Design review of the part built by this model. Coordinates are the model's own, in mm. A direction names the side the tool comes from. Give positions to 0.01 mm unless a question says otherwise; leave off trailing zeros. Loops run counter-clockwise (first coordinate to the right, second up) from the corner with the lowest first, then second, coordinate; pieces in that order, holes last. Notation, with made-up numbers: M 2.25,68.5 L 44.25,68.5 A20 cw 44.25,72.5 Z; hole C -2,-10.5 d6. An arc over 180 degrees is marked long. Use a Markdown table: item, result. Add a question column.
(1) Add section D-D, the plane x = -16.5. Give the boundary of the cut face in (y, z).
(2) For faces 4 (the face through (-5, 12.5, 0)), 5 (the face through (78.74, 18.78, -0.17)), list the 3-axis set-ups (+Z, -Z, +X, -X, +Y, -Y) from which the entire face can be reached by the end or side of a thin tool; tool diameter is ignored.
(3) Add section B-B, the plane x = 0. Give the boundary of the cut face in (y, z), then the cut area to 3 significant figures.
(4) For probe 1 along X at (y, z) = (28.75, 0); probe 2 along Y at (x, z) = (-37.5, 6.25); probe 3 along X at (y, z) = (18, 0), list the stretches that pass through material, from the lowest coordinate up.
(5) Add section A-A, the plane z = 0. Give the boundary of the cut face in (x, y).
(6) Add section C-C, the plane y = 29.5. Give the boundary of the cut face in (x, z).
(7) Draft analysis for pull direction Z (two halves, no side actions). For faces 1 (the face through (-58.42, 6.16, 0.17)), 2 (the face through (9, 10, -7.62)), 3 (the face through (2.52, 31.84, -0.33)), state which applies: pulls with the +Z half, pulls with the -Z half, needs draft (parallel to the pull), parting line crosses it, or undercut.
(8) Insertion check: pin 1 Ø1 at (y, z) = (23, -4) entering from +X; pin 2 Ø2 at (y, z) = (7.5, 0.5) entering from -X; pin 3 Ø1 at (y, z) = (31.5, -1.5) entering from +X; pin 4 Ø4 at (y, z) = (21.5, -0.5) entering from -X. Each pin has a flat end and moves straight along its axis. Give the tip position at first contact, or say it passes through.
```python
from build123d import *

# Parameters (mm, degrees)
BOSS_EXTRUDE1_DEPTH     = 38.1
SKETCH4_R               = 2.54
CUT_EXTRUDE3_DEPTH      = 88.804680969
CUT_EXTRUDE4_DEPTH      = 6.35
CUT_EXTRUDE4_DEPTH_BACK = 6.550000108


with BuildPart() as part:
    # Sketch3 → Boss-Extrude1 (new body)
    with BuildSketch(Plane(origin=(0, 0, 0), x_dir=(1, 0, 0), z_dir=(0, 1, 0))):
        with BuildLine():
            Line((-50.8, 7.62), (71.12, 7.62))
            ThreePointArc((71.12, 7.62), (78.74, 0), (71.12, -7.62))
            Line((71.12, -7.62), (-50.8, -7.62))
            ThreePointArc((-50.8, -7.62), (-58.42, 0), (-50.8, 7.62))
        make_face()
    extrude(amount=BOSS_EXTRUDE1_DEPTH)

    # Sketch4 → Cut-Extrude3 (cut, through all)
    with BuildSketch(Plane(origin=(0, 38.1, 0), x_dir=(1, 0, 0), z_dir=(0, 1, 0))):
        with Locations(Location((-50.8, 0, 0), (0, 0, 270))):
            Circle(SKETCH4_R)
        with Locations(Location((0, 0, 0), (0, 0, 270))):
            Circle(SKETCH4_R)
    extrude(amount=-CUT_EXTRUDE3_DEPTH, mode=Mode.SUBTRACT)

    # Sketch5 → Cut-Extrude4 (cut, two sides: drawn at the far end of the back side and taken through both)
    with BuildSketch(Plane(origin=(0, 19.05, 0), x_dir=(1, 0, 0), z_dir=(0, 1, 0)).offset(-CUT_EXTRUDE4_DEPTH_BACK)):
        with BuildLine():
            Line((25.4, 7.62), (-50.8, 7.62))
            ThreePointArc((-50.8, 7.62), (-58.42, 0), (-50.8, -7.62))
            Line((-50.8, -7.62), (0, -7.62))
            Line((0, -7.62), (50.8, -7.62))
            Line((50.8, -7.62), (50.8, 7.62))
            Line((50.8, 7.62), (25.4, 7.62))
        make_face()
    extrude(amount=CUT_EXTRUDE4_DEPTH + CUT_EXTRUDE4_DEPTH_BACK, mode=Mode.SUBTRACT)


solid = part.part
```
Established:
| question | item | result |
|---|---|---|
| 1 | outline | M 0,-7.62 L 12.5,-7.62 L 12.5,7.62 L 0,7.62 Z; M 25.4,-7.62 L 38.1,-7.62 L 38.1,7.62 L 25.4,7.62 Z |
| 2 | face 4 | +Z, -Z, -X |
| 2 | face 5 | +X, +Y, -Y |
| 3 | outline | M 0,-7.62 L 12.5,-7.62 L 12.5,-2.54 L 0,-2.54 Z; M 0,2.54 L 12.5,2.54 L 12.5,7.62 L 0,7.62 Z; M 25.4,-7.62 L 38.1,-7.62 L 38.1,-2.54 L 25.4,-2.54 Z; M 25.4,2.54 L 38.1,2.54 L 38.1,7.62 L 25.4,7.62 Z |
| 3 | area | 256 mm^2 |
| 4 | probe 1 | -58.42 to -53.34, -48.26 to -2.54, 2.54 to 78.74 |
| 4 | probe 2 | 0 to 12.5, 25.4 to 38.1 |
| 4 | probe 3 | 50.8 to 78.74 |
| 5 | outline | M -58.42,0 L -53.34,0 L -53.34,12.5 L -58.42,12.5 Z; M -58.42,25.4 L -53.34,25.4 L -53.34,38.1 L -58.42,38.1 Z; M -48.26,0 L -2.54,0 L -2.54,12.5 L -48.26,12.5 Z; M -48.26,25.4 L -2.54,25.4 L -2.54,38.1 L -48.26,38.1 Z; M 2.54,0 L 78.74,0 L 78.74,38.1 L 2.54,38.1 L 2.54,25.4 L 50.8,25.4 L 50.8,12.5 L 2.54,12.5 Z |
| 6 | outline | M -50.8,-7.62 L 71.12,-7.62 A7.62 ccw 71.12,7.62 L -50.8,7.62 A7.62 ccw Z; hole C -50.8,0 d5.08; hole C 0,0 d5.08 |
| 7 | face 1 | parting line crosses it |
| 7 | face 2 | pulls with the -Z half |
| 7 | face 3 | undercut |
| 8 | pin 1 | x = 77.89 |
| 8 | pin 2 | x = -58.42 |
| 8 | pin 3 | x = 78.67 |
| 8 | pin 4 | x = 50.8 |
